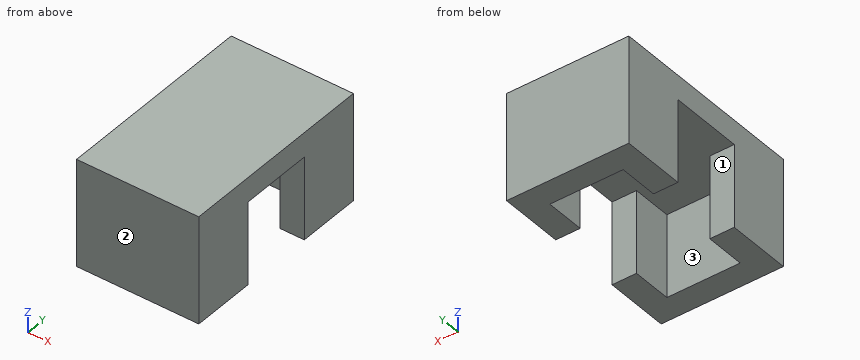
from build123d import *

# Parameters (mm, degrees)
F1_DEPTH = 6.8
F3_DEPTH = 2


with BuildPart() as f1:
    # F0 (on Top) → F1 (new body)
    with BuildSketch(Plane.XY):
        Polygon((-5, 5.236), (-5, 0), (-3, 0), (-3, 3.236), (0, 3.236), (3, 3.236), (3, 0), (5, 0), (5, 5.236), (0, 5.236), align=None)
    extrude(amount=F1_DEPTH)



with BuildPart() as f1b:
    # F0 (on Top) → F1, piece 2 (new body)
    with BuildSketch(Plane.XY):
        Polygon((-3, -6), (-5, -6), (-5, -11.236), (0, -11.236), (5, -11.236), (5, -6), (3, -6), (3, -9.236), (0, -9.236), (-3, -9.236), align=None)
    extrude(amount=F1_DEPTH)


with BuildPart() as f1_1:
    add(f1.part)

    add(f1b.part)  # F3 merges F1b
    # F2 (on face) → F3 (join)
    with BuildSketch(Plane.XY.offset(6.8)):
        Polygon((-3, 0), (-5, 0), (-5, -11.236), (5, -11.236), (5, 0), (3, 0), (3, 3.236), (-3, 3.236), align=None)
        Polygon((5, 5.236), (-5, 5.236), (-5, 0), (-3, 0), (-3, 3.236), (3, 3.236), (3, 0), (5, 0), align=None)
    extrude(amount=F3_DEPTH)


solid = f1_1.part
Can you work these out from the model? Positions are in its coordinate system, mm. Face numbers are marked on the shaded views. A direction names the side the tool comes from. Coordinates: 2 decimals unless noted, no trailing zeros. Write each loop counter-clockwise with the first axis right and the second up, starting at its lowest first coordinate (ties: lowest second). Pieces come first, ordered by that corner, then holes. Notation, with made-up numbers: (10, -4.75) - (33, -4.75) arc R13 cw to (33, 20.25) - close; hole circle Ø4 at (28.25, 61.25). An arc over 180 degrees is marked (long way). Return JSON: item names as keys, results as strings. Group by question number.
Item 1: If we section it at A-A (z = 6.25): Write out the boundary of the cut face in (x, y).
Item 2: If we section it at C-C (x = 0): Write out the boundary of the cut face in (y, z), then the cut area to 3 significant figures.
Item 3: Which directions (+Z, -Z, +X, -X, +Y, -Y) give clear straight access to the entire face, cutting with the end or side of a thin tool? Please do the marked faces 1, 2 and 3.
Item 4: Please list where these lines run through material, in increasing order: probe 1 along Y at (x, z) = (3.75, 3); probe 2 along Y at (x, z) = (-1, 1.5); probe 3 along X at (y, z) = (-7.5, 3).
Item 5: If we section it at B-B (y = -7): Write out the boundary of the cut face in (x, z), then the cut area to 3 significant figures.
Item 6: If we section it at D-D (y = -4.5): Write out the boundary of the cut face in (x, z), then the cut area to 3 significant figures.
Return value:
{
 "1": {"outline": "(-5, -11.24) - (5, -11.24) - (5, -6) - (3, -6) - (3, -9.24) - (-3, -9.24) - (-3, -6) - (-5, -6) - close; (-5, 0) - (-3, 0) - (-3, 3.24) - (3, 3.24) - (3, 0) - (5, 0) - (5, 5.24) - (-5, 5.24) - close"},
 "2": {"outline": "(-11.24, 0) - (-9.24, 0) - (-9.24, 6.8) - (3.24, 6.8) - (3.24, 0) - (5.24, 0) - (5.24, 8.8) - (-11.24, 8.8) - close", "area": "60.1 mm^2"},
 "3": {"face 1": "-Z, +X, -X", "face 2": "+Z, -Z, +X, -X, -Y", "face 3": "-Z"},
 "4": {"probe 1": "y = -11.24 to -6, 0 to 5.24", "probe 2": "y = -11.24 to -9.24, 3.24 to 5.24", "probe 3": "x = -5 to -3, 3 to 5"},
 "5": {"outline": "(-5, 0) - (-3, 0) - (-3, 6.8) - (3, 6.8) - (3, 0) - (5, 0) - (5, 8.8) - (-5, 8.8) - close", "area": "47.2 mm^2"},
 "6": {"outline": "(-5, 6.8) - (5, 6.8) - (5, 8.8) - (-5, 8.8) - close", "area": "20.0 mm^2"}
}
